```python
from build123d import *

# Parameters (mm, degrees)
F0_R     = 3
F0_R_2   = 0.715
F1_DEPTH = 5.67
F2_DEPTH = 6.15
F3_DEPTH = 10.58
F4_DEPTH = 2.25
F5_DEPTH = 0.91


with BuildPart() as f1:
    # F0 (on Top) → F1 (new body)
    with BuildSketch(Plane.XY):
        with BuildLine():
            ThreePointArc((4.038266955, -6.32), (6.5778796798, -3.6029847236), (7.5, 0))
            ThreePointArc((7.5, 0), (-3.6029847236, 6.5778796798), (-4.038266955, -6.32))
            Line((-4.038266955, -6.32), (-3.59, -6.32))
            Line((-3.59, -6.32), (3.59, -6.32))
            Line((3.59, -6.32), (4.038266955, -6.32))
        make_face()
        Circle(F0_R, mode=Mode.SUBTRACT)
        Circle(F0_R)
        Circle(F0_R_2, mode=Mode.SUBTRACT)
        with BuildLine():
            Line((-3.59, -6.32), (-3.59, -6.5849753227))
            ThreePointArc((-3.59, -6.5849753227), (0, -7.5), (3.59, -6.5849753227))
            Line((3.59, -6.5849753227), (3.59, -6.32))
            Line((3.59, -6.32), (-3.59, -6.32))
        make_face()
        Circle(F0_R_2)
        with BuildLine():
            ThreePointArc((3.59, -6.5849753227), (3.8164338282, -6.4563792357), (4.038266955, -6.32))
            Line((4.038266955, -6.32), (3.59, -6.32))
            Line((3.59, -6.32), (3.59, -6.5849753227))
        make_face()
        with BuildLine():
            Line((-3.59, -6.32), (-4.038266955, -6.32))
            ThreePointArc((-4.038266955, -6.32), (-3.8164338282, -6.4563792357), (-3.59, -6.5849753227))
            Line((-3.59, -6.5849753227), (-3.59, -6.32))
        make_face()
    extrude(amount=F1_DEPTH)

    # F0 (on Top) → F2 (join)
    with BuildSketch(Plane.XY):
        Circle(F0_R)
        Circle(F0_R_2, mode=Mode.SUBTRACT)
        Circle(F0_R_2)
    extrude(amount=F2_DEPTH)

    # F0 (on Top) → F3 (join)
    with BuildSketch(Plane.XY):
        Circle(F0_R_2)
    extrude(amount=F3_DEPTH)

    # F0 (on Top) → F4 (join)
    with BuildSketch(Plane.XY):
        with BuildLine():
            ThreePointArc((4.038266955, -6.32), (6.5778796798, -3.6029847236), (7.5, 0))
            ThreePointArc((7.5, 0), (-3.6029847236, 6.5778796798), (-4.038266955, -6.32))
            Line((-4.038266955, -6.32), (-3.59, -6.32))
            Line((-3.59, -6.32), (3.59, -6.32))
            Line((3.59, -6.32), (4.038266955, -6.32))
        make_face()
        Circle(F0_R, mode=Mode.SUBTRACT)
        Circle(F0_R)
        Circle(F0_R_2, mode=Mode.SUBTRACT)
        Circle(F0_R_2)
    extrude(amount=-F4_DEPTH)

    # F0 (on Top) → F5 (join)
    with BuildSketch(Plane.XY):
        with BuildLine():
            Line((-3.59, -6.32), (-3.59, -6.5849753227))
            ThreePointArc((-3.59, -6.5849753227), (0, -7.5), (3.59, -6.5849753227))
            Line((3.59, -6.5849753227), (3.59, -6.32))
            Line((3.59, -6.32), (-3.59, -6.32))
        make_face()
        with BuildLine():
            ThreePointArc((3.59, -6.5849753227), (0, -7.5), (-3.59, -6.5849753227))
            Line((-3.59, -6.5849753227), (-3.59, -14.931))
            Line((-3.59, -14.931), (3.59, -14.931))
            Line((3.59, -14.931), (3.59, -6.5849753227))
        make_face()
    extrude(amount=-F5_DEPTH)


solid = f1.part
```
Work out the finished part from the listing and answer in its coordinate system (mm). A direction names the side the tool comes from. Coordinates: 2 decimals unless noted, no trailing zeros. Loops run counter-clockwise (first coordinate to the right, second up) from the corner with the lowest first, then second, coordinate; pieces in that order, holes last. Notation, with made-up numbers: M 56,64 L 73,64 A20 ccw 73,91 Z; hole C 79.5,-31 d5. An arc over 180 degrees is marked long. Use CSV: the item, a comma, the result in double quotes. Start each with the question number.
(1) For faces 1 (the face through (0, -11, -0.91)), 2 (the face through (3.2, 0.1, 5.67)), 3 (the face through (-0.1, -14.931, -0.4)), determine the directions among +Z, -Z, +X, -X, +Y, -Y from which every point of the face is accessible in a straight line to the end or side of a thin tool.
(2) Find section D-D, the plane x = 2.75. Give the vertices of the cut face in (y, z), then the cut area to 3 significant figures.
(3) Find section A-A, the plane x = 0. Give the vertices of the cut face in (y, z) (3 decimals).
(4) Given pin 1 Ø8 at (x, y) = (0.5, -12.5) entering from +Z; pin 2 Ø8 at (x, y) = (0, -10.5) entering from -Z; pin 3 Ø4 at (x, z) = (-2.5, 0) entering from +Y, each flat-ended and moving along its own axis, determine where each tip first touches the part or whether it passes through.
(5) Consider line 1 (Z direction, x = -2.5, y = -9.5); line 2 (Z direction, x = 6.5, y = -0.75); line 3 (X direction, y = -6.75, z = -0.5). Determine where each line is inside the solid, lowest interval first.
(6) Find section B-B, the plane z = 4.5. Give the vertices of the cut face in (x, y).
(7) Find section C-C, the plane y = -2.75. Give the vertices of the cut face in (x, z), then the cut area to 3 significant figures.
Recorded:
1,face 1,"-Z, +X, -X, -Y"
1,face 2,"+Z"
1,face 3,"+Z, -Z, +X, -X, -Y"
2,outline,"M -14.93,-0.91 L -6.32,-0.91 L -6.32,-2.25 L 6.98,-2.25 L 6.98,5.67 L 1.2,5.67 L 1.2,6.15 L -1.2,6.15 L -1.2,5.67 L -6.98,5.67 L -6.98,0 L -14.93,0 Z"
2,area,"118 mm^2"
3,outline,"M -14.931,-0.91 L -6.32,-0.91 L -6.32,-2.25 L 7.5,-2.25 L 7.5,5.67 L 3,5.67 L 3,6.15 L 0.715,6.15 L 0.715,10.58 L -0.715,10.58 L -0.715,6.15 L -3,6.15 L -3,5.67 L -7.5,5.67 L -7.5,0 L -14.931,0 Z"
4,pin 1,"stops at z = 0"
4,pin 2,"stops at z = -0.91"
4,pin 3,"stops at y = 7.48"
5,line 1,"z = -0.91 to 0"
5,line 2,"z = -2.25 to 5.67"
5,line 3,"x = -3.59 to 3.59"
6,outline,"C 0,0 d15"
7,outline,"M -6.98,-2.25 L 6.98,-2.25 L 6.98,5.67 L 1.2,5.67 L 1.2,6.15 L -1.2,6.15 L -1.2,5.67 L -6.98,5.67 Z"
7,area,"112 mm^2"
